from build123d import *

# Parameters (mm, degrees)
F0_W           = 9.5
F0_H           = 42.5
F1_DEPTH       = 4.5
F3_D           = 3.1
F3_CBORE_D     = 5.9
F3_CBORE_DEPTH = 2.2
F4_W           = 11
F4_H           = 29.5
F5_DEPTH       = 4
F7_D           = 2.83
F8_W           = 7
F8_H           = 13
F9_DEPTH       = 25
F10_T1_DEPTH   = 4.5
F11_R          = 2
F12_SIZE       = 5
F13_R          = 1


# Not quite as in the source:
# - a fillet or chamfer that OpenCascade refuses, or shapes differently, is made with other operations: its cross-section is extruded or revolved along the edge and cut away or added


with BuildPart() as f1:
    # F0 (on Top) → F1 (new body)
    with BuildSketch(Plane.XY):
        with Locations((-4.75, 21.25)):
            Rectangle(F0_W, F0_H)
    extrude(amount=F1_DEPTH)

    # F3 (through all)
    with Locations(Plane.XY.offset(4.5)):
        with Locations((-5.5, 36.5), (-5.5, 5.5)):
            CounterBoreHole(F3_D / 2, F3_CBORE_D / 2, F3_CBORE_DEPTH)

    # F4 (on Right) → F5 (join)
    with BuildSketch(Plane.YZ):
        with Locations((48, -10.25)):
            Rectangle(F4_W, F4_H)
    extrude(amount=-F5_DEPTH)

    # F7 (through all)
    with Locations(Plane.YZ):
        with Locations((48, -3.3), (48, -22.3)):
            Hole(F7_D / 2)

    # F8 (on face) → F9 (cut)
    with BuildSketch(Plane.YZ):
        with Locations((48, -12.5)):
            Rectangle(F8_W, F8_H)
    extrude(amount=-F9_DEPTH, mode=Mode.SUBTRACT)

    # F10: fillet of radius 5 on 1 edges, made by hand

    # F10_s2 → F10_t1 (join)
    with BuildSketch(Plane.XY):
        with BuildLine():
            ThreePointArc((-9.0009656854, 42.4996), (-5.4644660941, 43.9644660941), (-3.9996, 47.5009656854))
            Line((-3.9996, 47.5009656854), (-3.4994634315, 47.5009656854))
            ThreePointArc((-3.4994634315, 47.5009656854), (-3.4998634315, 45.0004828427), (-3.4998634315, 42.5))
            Line((-3.4998634315, 42.5), (-4, 41.9998634315))
            ThreePointArc((-4, 41.9998634315), (-6.5004828427, 41.9998634315), (-9.0009656854, 41.9994634315))
            Line((-9.0009656854, 41.9994634315), (-9.0009656854, 42.4996))
        make_face()
    extrude(amount=F10_T1_DEPTH)

    # F11
    f11_edges = [f1.edges().sort_by_distance(p)[0] for p in [
        (-2, 53.5, 4.5),
        (-2, 53.5, -25),
        (-2, 42.5, -25),
        (-9.5, 42.5, 2.25),
    ]]
    fillet(f11_edges, radius=F11_R)

    # F12
    f12_edges = [f1.edges().sort_by_distance(p)[0] for p in [
        (0, 0, 2.25),
    ]]
    chamfer(f12_edges, length=F12_SIZE)

    # F13
    f13_edges = [f1.edges().sort_by_distance(p)[0] for p in [
        (-2, 44.5, -6),
        (-2, 51.5, -6),
        (-2, 44.5, -19),
        (-2, 51.5, -19),
        (-9.5, 0, 2.25),
    ]]
    fillet(f13_edges, radius=F13_R)


solid = f1.part
Here's how the part is built. I have some questions about the finished solid (model axes, mm). A direction names the side the tool comes from. Round coordinates to 2 decimals unless told otherwise and drop trailing zeros. Loops run counter-clockwise (first coordinate to the right, second up) from the corner with the lowest first, then second, coordinate; pieces in that order, holes last.
1. If we section it at D-D on x = -5.75: Write out the boundary of the cut face in (y, z), plus the area to 3 significant figures.
Answer list:
outline: (0, 0) - (3.97, 0) - (3.97, 2.3) - (2.56, 2.3) - (2.56, 4.5) - (0, 4.5) - close; (7.03, 0) - (34.97, 0) - (34.97, 2.3) - (33.56, 2.3) - (33.56, 4.5) - (8.44, 4.5) - (8.44, 2.3) - (7.03, 2.3) - close; (38.03, 0) - (43.7, 0) - (43.7, 4.5) - (39.44, 4.5) - (39.44, 2.3) - (38.03, 2.3) - close
area: 157 mm2
2. If I drill on line 1 along Z through (x, y) = (-2.65, 48) (3 decimals); line 2 along Y through (x, z) = (-5.5, 3.4); line 3 along Y through (x, z) = (-5.5, 1.35), over which ranges is the centre line in solid material (lowest first)?
Answer list:
line 1: z = -25 to -23.715, -20.885 to -19, -6 to -4.715, -1.885 to 4.5
line 2: y = 0 to 2.55, 8.45 to 33.55, 39.45 to 43.93
line 3: y = 0 to 3.95, 7.05 to 34.95, 38.05 to 43.93
3. If we section it at C-C on y = 48: Write out the boundary of the cut face in (x, z) (3 decimals), plus the area to 3 significant figures.
Answer list:
outline: (-4, -25) - (0, -25) - (0, -23.715) - (-4, -23.715) - close; (-4, -20.885) - (0, -20.885) - (0, -19) - (-4, -19) - close; (-4, -6) - (0, -6) - (0, -4.715) - (-4, -4.715) - close; (-4, -1.885) - (0, -1.885) - (0, 4.5) - (-4, 4.5) - close
area: 43.4 mm2
4. For P1, Ø9, axis at y = 48.5, z = -3, coming from the -X side; P2, Ø4, axis at x = -5.5, y = 5.5, coming from the -Z side; P3, Ø5, axis at x = -5.5, y = 36.5, coming from the +Z side, each with a flat end and sliding along its axis, tell me the tip position at first contact or that it passes through.
Answer list:
P1: stops at x = -4.59
P2: stops at z = 0
P3: stops at z = 2.3
5. We'd pull the mould along Y, two halves only. Please class faces 4 (the face through (-2.03, 43.1, -24.43)), 5 (the face through (-2.03, 46.69, -3.84)), 6 (the face through (-9.5, 21, 2)): +Y half, -Y half, draft (parallel to the pull), parting line (faces both ways), or undercut.
Answer list:
face 4: -Y half
face 5: undercut
face 6: draft
6. Which directions (+Z, -Z, +X, -X, +Y, -Y) give clear straight access to the entire face, cutting with the end or side of a thin tool? Please do faces 1 (the face through (-2.028, 44.801, -18.715)), 2 (the face through (-2, 42.5, -12)), 3 (the face through (-2.686, 37.386, 3.415)).
Answer list:
face 1: +X, -X
face 2: -Z, +X, -X, -Y
face 3: +Z
7. If we section it at A-A on z = -9.5: Write out the boundary of the cut face in (x, y).
Answer list:
outline: (-4, 42.5) - (0, 42.5) - (0, 44.5) - (-4, 44.5) - close; (-4, 51.5) - (0, 51.5) - (0, 53.5) - (-4, 53.5) - close
8. If we section it at B-B on y = 5.5: Write out the boundary of the cut face in (x, z), plus the area to 3 significant figures.
Answer list:
outline: (-9.5, 0) - (-7.05, 0) - (-7.05, 2.3) - (-8.45, 2.3) - (-8.45, 4.5) - (-9.5, 4.5) - close; (-3.95, 0) - (0, 0) - (0, 4.5) - (-2.55, 4.5) - (-2.55, 2.3) - (-3.95, 2.3) - close
area: 22.6 mm2
